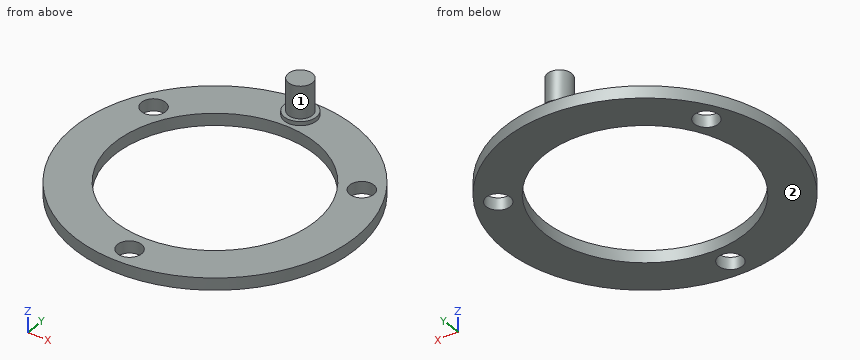
Autodesk Inventor part; units mm, degrees
ref_plane "YZ Plane" through (0, 0, 0) normal (1, 0, 0) x (0, 1, 0)
ref_plane "XZ Plane" through (0, 0, 0) normal (0, 1, 0) x (-1, 0, 0)
ref_plane "XY Plane" through (0, 0, 0) normal (0, 0, 1) x (1, 0, 0)
sketch "Sketch1" plane through (0, 0, 0) normal (0, 0, 1) x (1, 0, 0)
  circle A0 centre (0, 0) radius 30 construction
  line L0 (0, 0) -> (0, 7.5) construction
  line L1 (0, 7.5) -> (10, 7.5) construction
  line L2 (10, 7.5) -> (10, 0) construction
  line L3 (10, 0) -> (0, 0) construction
  line L4 (0, 0) -> (-10, 0) construction
  line L5 (-10, 0) -> (-10, 7.5) construction
  line L6 (-10, 7.5) -> (0, 7.5) construction
  line L7 (-10, 0) -> (-10, -7.5) construction
  line L8 (-10, -7.5) -> (10, -7.5) construction
  line L9 (10, -7.5) -> (10, 0) construction
  circle A1 centre (-15.5891, 25.6316) radius 10 construction
  circle A2 centre (0, 0) radius 35
  circle A3 centre (0, 0) radius 25
  line L10 (0, 0) -> (-31.8198, 31.8198) construction
  circle A4 centre (0, 0) radius 45 construction
  line L11 (0, 0) -> (0, 45) construction
  circle A5 centre (0, 0) radius 40 construction
  circle A6 centre (-40, 0) radius 5 construction
  circle A7 centre (-31.8198, 31.8198) radius 10 construction
  line L12 (-31.8198, 31.8198) -> (-31.8198, -24.2384) construction
  line L13 (-31.8198, -24.2384) -> (-31.8198, -31.8198) construction
  circle A8 centre (-31.8198, -31.8198) radius 10 construction
  line L14 (-15, -20) -> (-15, -31.6228) construction
  line L15 (15, -20) -> (15, -31.6228) construction
  line L16 (-31.8198, 31.8198) -> (24.2384, 31.8198) construction
  line L17 (24.2384, 31.8198) -> (31.8198, 31.8198) construction
  line L18 (31.8198, 31.8198) -> (31.8198, -31.8198) construction
  line L19 (31.8198, -31.8198) -> (-31.8198, -31.8198) construction
  circle A9 centre (31.8198, 31.8198) radius 10 construction
  circle A10 centre (31.8198, -31.8198) radius 10 construction
  circle A11 centre (0, 40) radius 5 construction
  line L20 (0, 0) -> (40, 0) construction
  line L21 (0, 0) -> (0, -40) construction
  circle A12 centre (40, 0) radius 5 construction
  circle A13 centre (0, -40) radius 5 construction
  line L22 (50, 50) -> (50, -50) construction
  line L23 (50, -50) -> (-50, -50) construction
  line L24 (-50, -50) -> (-50, 50) construction
  line L25 (-50, 50) -> (50, 50) construction
  circle A14 centre (0, 30) radius 3
  point P0 (0, 50)
  dimension "d9" = 80
  dimension "d0" = 60
  dimension "d1" = 20
  dimension "d2" = 15
  dimension "d3" = 20
  dimension "d4" = 5
  dimension "d5" = 5
  dimension "d6" = 90
  dimension "d7" = 45
  dimension "d10" = 10
  dimension "d12" = 20
  dimension "d13" = 15
  dimension "d14" = 100
  dimension "d15" = 6
extrude "Extrusion1" add sketch "Sketch1" along normal blind 3
sketch "Sketch2" plane through (0, 0, 0) normal (0, 0, -1) x (-1, 0, 0)
  circle A0 centre (0, 30) radius 3
extrude "Extrusion2" add sketch "Sketch2" against normal blind 12
sketch "Sketch3" plane through (0, 0, 3) normal (0, 0, 1) x (1, 0, 0)
  circle A0 centre (0, 30) radius 3
  circle A1 centre (0, 30) radius 4
  dimension "d20" = 8
extrude "Extrusion3" add sketch "Sketch3" along normal blind 1
sketch "Sketch4" plane through (0, 0, 3) normal (0, 0, 1) x (1, 0, 0)
  circle A0 centre (0, 0) radius 25
  circle A1 centre (0, 0) radius 35
  line L0 (0, 0) -> (0, -25) construction
  line L1 (0, -25) -> (0, -35) construction
  circle A2 centre (0, -30) radius 3
  dimension "d23" = 6
extrude "Extrusion4" cut sketch "Sketch4" against normal blind 10 contours A2
pattern_circular "Circular Pattern1" count 3 over 360 about axis through (0, 0, -10) along (0, 0, 1) of "Extrusion4"
properties part number "Ring1"
Geometry check sheet. Reference: the model listing, model coordinates, mm. Face numbers are marked on the shaded views. A direction names the side the tool comes from. Round coordinates to 2 decimals unless told otherwise and drop trailing zeros. Loops run counter-clockwise (first coordinate to the right, second up) from the corner with the lowest first, then second, coordinate; pieces in that order, holes last. Notation, with made-up numbers: (20, 73) -> (69, 73) arc R36 ccw to (69, 109) -> close; hole circle Ø7 at (-2.75, 8). An arc over 180 degrees is marked (long way). Answer as a JSON object with one key per item and string values. Group by question number.
Item 1: Depth check by flat-ended pin: pin 1 Ø2 at (y, z) = (7.5, 2) entering from -X; pin 2 Ø3.5 at (x, y) = (0, -30) entering from -Z; pin 3 Ø1.5 at (y, z) = (27, 10.5) entering from -X. Enter the tip coordinate at first touch or a pass-through.
Item 2: Set-up check for the marked faces 1 and 2: record each of +Z, -Z, +X, -X, +Y, -Y from which the full face is reachable in a straight line by a thin tool's end or side.
Item 3: Cross-section at D-D, the plane x = 9. Record the cut outline in (y, z).
Item 4: Cross-section at C-C, the plane y = 15. Record the cut outline in (x, z), plus the area to 3 significant figures.
Item 5: Cross-section at B-B, the plane x = 0. Record the cut outline in (y, z).
Item 6: Thickness scan on line 1 along Y through (x, z) = (0, 2.3); line 2 along Z through (x, y) = (-9.5, 29); line 3 along Y through (x, z) = (-26, 2.25). Record the ranges inside material, lowest first.
Item 7: Cross-section at A-A, the plane y = 0. Record the cut outline in (x, z), plus the area to 3 significant figures.
Determined:
{
 "1": {"pin 1": "stops at x = -34.39", "pin 2": "passes through", "pin 3": "stops at x = -1.98"},
 "2": {"face 1": "+Z", "face 2": "-Z, +X, -X, +Y, -Y"},
 "3": {"outline": "(-33.82, 0) -> (-23.32, 0) -> (-23.32, 3) -> (-33.82, 3) -> close; (23.32, 0) -> (33.82, 0) -> (33.82, 3) -> (23.32, 3) -> close"},
 "4": {"outline": "(-31.62, 0) -> (-28.98, 0) -> (-28.98, 3) -> (-31.62, 3) -> close; (-22.98, 0) -> (-20, 0) -> (-20, 3) -> (-22.98, 3) -> close; (20, 0) -> (22.98, 0) -> (22.98, 3) -> (20, 3) -> close; (28.98, 0) -> (31.62, 0) -> (31.62, 3) -> (28.98, 3) -> close", "area": "33.7 mm²"},
 "5": {"outline": "(-35, 0) -> (-33, 0) -> (-33, 3) -> (-35, 3) -> close; (-27, 0) -> (-25, 0) -> (-25, 3) -> (-27, 3) -> close; (25, 0) -> (35, 0) -> (35, 3) -> (34, 3) -> (34, 4) -> (33, 4) -> (33, 12) -> (27, 12) -> (27, 4) -> (26, 4) -> (26, 3) -> (25, 3) -> close"},
 "6": {"line 1": "y = -35 to -33, -27 to -25, 25 to 35", "line 2": "z = 0 to 3", "line 3": "y = -23.43 to 12, 18 to 23.43"},
 "7": {"outline": "(-35, 0) -> (-25, 0) -> (-25, 3) -> (-35, 3) -> close; (25, 0) -> (35, 0) -> (35, 3) -> (25, 3) -> close", "area": "60.0 mm²"}
}
